Check sheet for the modelled part. Datum: model origin and axes. Units: mm. A direction names the side the tool comes from. Give positions to 0.01 mm unless a question says otherwise; leave off trailing zeros. Loops run counter-clockwise (first coordinate to the right, second up) from the corner with the lowest first, then second, coordinate; pieces in that order, holes last. Notation, with made-up numbers: (80, 56) -> (114, 56) arc R21 ccw to (114, 67) -> close; hole circle Ø6 at (-25, 89.5). An arc over 180 degrees is marked (long way). Write each question's results on one line, items separated by ' | '. Start each with the question number.
Item 1: Scan lines: line 1 along X through (y, z) = (13, 0.25); line 2 along Y through (x, z) = (-10, 0.4); line 3 along X through (y, z) = (-8, 1.5). Record each from-to range of solid material in increasing order.
Item 2: Mould release check, pull along X, two halves, no side actions. Record for faces 1 (the face through (14.147, -17.717, 0.792)), 2 (the face through (-14.85, -18.43, 0.79)), 3 (the face through (16.5, 0, 1)): pulls with the +X half, pulls with the -X half, needs draft (parallel to the pull), parting line crosses it, or undercut.
Item 3: Access from +Z, -Z, +X, -X, +Y, -Y to the whole of each face (thin tool, end or side, straight path). Record for faces 4 (the face through (0, -19, 1)), 5 (the face through (14.85, 18.43, 0.79)).
Item 4: Cross-section at C-C on x = 4. Enter the section's corners in (y, z), then the cut area to 3 significant figures.
Item 5: Cross-section at B-B on z = 0.95. Enter the section's corners in (x, y), then the cut area to 3 significant figures.
Item 6: Cross-section at A-A on y = -13. Enter the section's corners in (x, z).
from build123d import *

# Parameters (mm, degrees)
AUFSATZ_LINEAR_AUSTRAGEN1_DEPTH = 1.6
FASE1_SIZE                      = 0.2


with BuildPart() as part:
    # Skizze1 → Aufsatz-Linear austragen1 (new body)
    with BuildSketch(Plane(origin=(0, 0, 0), x_dir=(0, 1, 0), z_dir=(0, 0, 1))):
        with BuildLine():
            Line((-20, -11), (-20, 11))
            ThreePointArc((-20, 11), (-18.389087297, 14.889087297), (-14.5, 16.5))
            Line((-14.5, 16.5), (14.5, 16.5))
            ThreePointArc((14.5, 16.5), (18.389087297, 14.889087297), (20, 11))
            Line((20, 11), (20, -11))
            ThreePointArc((20, -11), (18.389087297, -14.889087297), (14.5, -16.5))
            Line((14.5, -16.5), (-14.5, -16.5))
            ThreePointArc((-14.5, -16.5), (-18.389087297, -14.889087297), (-20, -11))
        make_face()
        with BuildLine():
            Line((-14.5, -15.5), (14.5, -15.5))
            ThreePointArc((14.5, -15.5), (17.681980515, -14.181980515), (19, -11))
            Line((19, -11), (19, 11))
            ThreePointArc((19, 11), (17.681980515, 14.181980515), (14.5, 15.5))
            Line((14.5, 15.5), (-14.5, 15.5))
            ThreePointArc((-14.5, 15.5), (-17.681980515, 14.181980515), (-19, 11))
            Line((-19, 11), (-19, -11))
            ThreePointArc((-19, -11), (-17.681980515, -14.181980515), (-14.5, -15.5))
        make_face(mode=Mode.SUBTRACT)
    extrude(amount=AUFSATZ_LINEAR_AUSTRAGEN1_DEPTH)

    # Fase1
    fase1_edges = [part.edges().sort_by_distance(p)[0] for p in [
        (16.5, 0, 0),
        (14.889087297, -18.389087297, 0),
        (0, -20, 0),
        (-14.889087297, -18.389087297, 0),
        (14.889087297, -18.389087297, 1.6),
        (16.5, 0, 1.6),
        (14.889087297, 18.389087297, 1.6),
        (0, 20, 1.6),
        (14.181980515, 17.681980515, 0),
        (0, 19, 0),
        (-14.181980515, 17.681980515, 0),
        (-15.5, 0, 0),
        (-14.889087297, 18.389087297, 1.6),
        (-14.181980515, -17.681980515, 0),
        (0, -19, 0),
        (14.181980515, -17.681980515, 0),
        (15.5, 0, 0),
        (14.181980515, 17.681980515, 1.6),
        (0, 19, 1.6),
        (-14.181980515, 17.681980515, 1.6),
        (-15.5, 0, 1.6),
        (-14.181980515, -17.681980515, 1.6),
        (0, -19, 1.6),
        (14.181980515, -17.681980515, 1.6),
        (-16.5, 0, 1.6),
        (15.5, 0, 1.6),
        (-14.889087297, -18.389087297, 1.6),
        (-16.5, 0, 0),
        (0, -20, 1.6),
        (-14.889087297, 18.389087297, 0),
        (0, 20, 0),
        (14.889087297, 18.389087297, 0),
    ]]
    chamfer(fase1_edges, length=FASE1_SIZE)


solid = part.part
Answer sheet:
1) line 1: x = -16.5 to -15.5, 15.5 to 16.5 | line 2: y = -20 to -19, 19 to 20 | line 3: x = -16.4 to -15.6, 15.6 to 16.4
2) face 1: undercut | face 2: pulls with the -X half | face 3: pulls with the +X half
3) face 4: +Z, -Z | face 5: +Z, -Z, +X, +Y
4) outline: (-20, 0.2) -> (-19.8, 0) -> (-19.2, 0) -> (-19, 0.2) -> (-19, 1.4) -> (-19.2, 1.6) -> (-19.8, 1.6) -> (-20, 1.4) -> close; (19, 0.2) -> (19.2, 0) -> (19.8, 0) -> (20, 0.2) -> (20, 1.4) -> (19.8, 1.6) -> (19.2, 1.6) -> (19, 1.4) -> close | area: 3.04 mm²
5) outline: (-16.5, -14.5) arc R5.5 ccw to (-11, -20) -> (11, -20) arc R5.5 ccw to (16.5, -14.5) -> (16.5, 14.5) arc R5.5 ccw to (11, 20) -> (-11, 20) arc R5.5 ccw to (-16.5, 14.5) -> close; hole (-15.5, -14.5) arc R4.5 ccw to (-11, -19) -> (11, -19) arc R4.5 ccw to (15.5, -14.5) -> (15.5, 14.5) arc R4.5 ccw to (11, 19) -> (-11, 19) arc R4.5 ccw to (-15.5, 14.5) -> close | area: 133 mm²
6) outline: (-16.5, 0.2) -> (-16.3, 0) -> (-15.7, 0) -> (-15.5, 0.2) -> (-15.5, 1.4) -> (-15.7, 1.6) -> (-16.3, 1.6) -> (-16.5, 1.4) -> close; (15.5, 0.2) -> (15.7, 0) -> (16.3, 0) -> (16.5, 0.2) -> (16.5, 1.4) -> (16.3, 1.6) -> (15.7, 1.6) -> (15.5, 1.4) -> close
